```python
from build123d import *

# Parameters (mm, degrees)
SKETCH1_W           = 100
SKETCH1_H           = 50
BOSS_EXTRUDE1_DEPTH = 5
CUT_EXTRUDE1_DEPTH  = 57.124860802
CUT_EXTRUDE2_DEPTH  = 57.124860802
BOSS_EXTRUDE2_DEPTH = 20


with BuildPart() as part:
    # Sketch1 → Boss-Extrude1 (new body)
    with BuildSketch(Plane.XY):
        Rectangle(SKETCH1_W, SKETCH1_H)
    extrude(amount=BOSS_EXTRUDE1_DEPTH)

    # Sketch2 → Cut-Extrude1 (cut, through all)
    with BuildSketch(Plane(origin=(0, 0, 0), x_dir=(-1, 0, 0), z_dir=(0, 0, -1))):
        Polygon((-50, 1.666666667), (-15, 25), (-50, 25), align=None)
        Polygon((50, 25), (15, 25), (50, 1.666666667), align=None)
    extrude(amount=-CUT_EXTRUDE1_DEPTH, mode=Mode.SUBTRACT)

    # Sketch3 → Cut-Extrude2 (cut, through all)
    with BuildSketch(Plane.XY.offset(5)):
        Polygon((-50, -3.333333333), (-15, 20), (15, 20), (50, -3.333333333), (50, -25), (-50, -25), align=None)
    extrude(amount=-CUT_EXTRUDE2_DEPTH, mode=Mode.SUBTRACT)

    # Sketch4 → Boss-Extrude2 (add)
    with BuildSketch(Plane.XY.offset(5)):
        Polygon((-50, 1.666666667), (-50, -3.333333333), (-15, 20), (15, 20), (50, -3.333333333), (50, 1.666666667), (15, 25), (-15, 25), align=None)
    extrude(amount=BOSS_EXTRUDE2_DEPTH)


solid = part.part
```
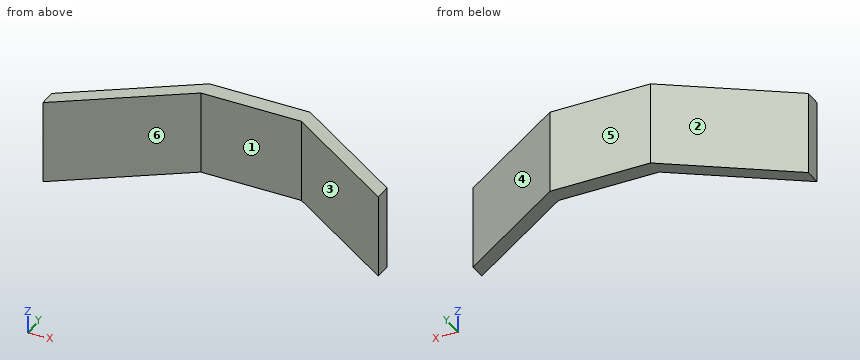
Source: CAD feature listing. Evaluate the final solid. Frame: model axes, mm. Face numbers are marked on the shaded views. A direction names the side the tool comes from. Give positions to 0.01 mm unless a question says otherwise; leave off trailing zeros. Order: outer loops, then holes, each group sorted by start corner. A loop starts at its lowest first (then second) coordinate and runs counter-clockwise, first axis right, second up.
(1) Section query B-B (z = 7.75). Return the cut outline in (x, y).
(2) Contact query for flat-ended pins moving along their axis: P1, Ø3, axis at x = 2.5, z = 4, coming from the -Y side; P2, Ø1.5, axis at y = 11, z = 15, coming from the +X side (3 decimals); P3, Ø2, axis at y = 12, z = 16.5, coming from the +X side; P4, Ø4, axis at x = 21, y = 14.5, coming from the -Z side. Output: stop coordinate, or through.
(3) Section query C-C (x = -24). Return the cut outline in (y, z).
(4) Section query A-A (y = 9). Return the cut outline in (x, z), plus the area to 3 significant figures.
(5) Section query D-D (y = 21.5). Return the cut outline in (x, z), plus the area to 3 significant figures.
(6) Material intervals for line 1 along X through (y, z) = (10, 18.75); line 2 along X through (y, z) = (-0.25, 4.25) (3 decimals); line 3 along Y through (x, z) = (13.5, 20.25), sorted ascending.
(7) Access query for the marked faces 1 and 2. Directions: +Z, -Z, +X, -X, +Y, -Y. A direction counts if a zero-diameter tool reaches every point of the face in a straight line with its end or side. Return the directions, or none.
(8) Pull-direction query (X, two-part tool) for the marked faces 3, 4, 5 and 6; classes: +X half, -X half, draft (parallel to the pull), parting line (faces both ways), or undercut.
Outcome:
1. outline: (-50, -3.33) - (-15, 20) - (15, 20) - (50, -3.33) - (50, 1.67) - (15, 25) - (-15, 25) - (-50, 1.67) - close
2. P1: stops at y = 20
2. P2: stops at x = 37.125
2. P3: stops at x = 36
2. P4: stops at z = 0
3. outline: (14, 0) - (19, 0) - (19, 25) - (14, 25) - close
4. outline: (-39, 0) - (-31.5, 0) - (-31.5, 25) - (-39, 25) - close; (31.5, 0) - (39, 0) - (39, 25) - (31.5, 25) - close
4. area: 375 mm2
5. outline: (-20.25, 0) - (20.25, 0) - (20.25, 25) - (-20.25, 25) - close
5. area: 1,010 mm2
6. line 1: x = -37.5 to -30, 30 to 37.5
6. line 2: x = -50 to -45.375, 45.375 to 50
6. line 3: y = 20 to 25
7. face 1: +Z, -Z, -Y
7. face 2: +Z, -Z, -X, +Y
8. face 3: undercut
8. face 4: +X half
8. face 5: draft
8. face 6: undercut
